The listing builds one solid part. Answer for the finished solid, in the listing's coordinates (mm). Round coordinates to 2 decimals unless told otherwise and drop trailing zeros. Write each loop counter-clockwise with the first axis right and the second up, starting at its lowest first coordinate (ties: lowest second). Pieces come first, ordered by that corner, then holes.
(1) A cutting plane is placed at A-A, the plane y = 0. Give the vertices of the cut face in (x, z), and give its area (3 significant figures).
(2) A cutting plane is placed at D-D, the plane z = 1.1. Give the number of separate pieces and of enclosed holes in the cut face, and give its area (3 significant figures).
(3) Each of these flat-tipped pins is pushed along its axis until it touches: pin 1 Ø1 at (x, z) = (22, 0.5) entering from +Y; pin 2 Ø3.5 at (x, y) = (-52.5, 0) entering from +Z. Where does it stop, or does it pass through?
(4) A cutting plane is placed at C-C, the plane y = 31.5. Give the vertices of the cut face in (x, z), and give its area (3 significant figures).
(5) Find the intervals of material crossed by probe 1 along Y at (x, z) = (-38, 1.4); probe 2 along Y at (x, z) = (19.5, 1.55); probe 3 along X at (y, z) = (25, 1.8), in increasing order.
from build123d import *

# Parameters (mm, degrees)
SKETCH_1_R          = 75
SKETCH_1_R_2        = 2
SKETCH_1_R_3        = 46
EXTRUDE_1_DEPTH     = 2
CUT_EXTRUDE_2_DEPTH = 10
SKETCH_5_R          = 1.65
CUT_EXTRUDE_3_DEPTH = 10
FILLET_2_R          = 2


with BuildPart() as part:
    # 草图1 → 凸台-拉伸1 (new body)
    with BuildSketch(Plane.XY):
        Circle(SKETCH_1_R)
        with Locations((-52.5, 0)):
            Circle(SKETCH_1_R_2, mode=Mode.SUBTRACT)
        with Locations((0, 52.5)):
            Circle(SKETCH_1_R_2, mode=Mode.SUBTRACT)
        with Locations((52.5, 0)):
            Circle(SKETCH_1_R_2, mode=Mode.SUBTRACT)
        with Locations((0, -52.5)):
            Circle(SKETCH_1_R_2, mode=Mode.SUBTRACT)
        Circle(SKETCH_1_R_3, mode=Mode.SUBTRACT)
    extrude(amount=EXTRUDE_1_DEPTH)

    # 草图3 → 切除-拉伸2 (cut)
    with BuildSketch(Plane.XY.offset(2)):
        with BuildLine():
            Line((-51.775970298, -18.553945664), (-61.172994758, -21.974182859))
            ThreePointArc((-61.172994758, -21.974182859), (-46.153503513, -45.769576287), (-22.484399296, -60.98730842))
            Line((-22.484399296, -60.98730842), (-19.064163111, -51.59028673))
            ThreePointArc((-19.064163111, -51.59028673), (-39.082362813, -38.698435587), (-51.775970298, -18.553945664))
        make_face()
        with BuildLine():
            Line((51.775970298, 18.553945664), (61.172994758, 21.974182859))
            ThreePointArc((61.172994758, 21.974182859), (46.153503513, 45.769576287), (22.484399296, 60.98730842))
            Line((22.484399296, 60.98730842), (19.064163111, 51.59028673))
            ThreePointArc((19.064163111, 51.59028673), (39.082362813, 38.698435587), (51.775970298, 18.553945664))
        make_face()
    extrude(amount=-CUT_EXTRUDE_2_DEPTH, mode=Mode.SUBTRACT)

    # 草图5 → 切除-拉伸3 (cut)
    with BuildSketch(Plane.XY.offset(2)):
        with Locations((-63.53412763, 21.527067294)):
            Circle(SKETCH_5_R)
        with Locations((-42.216475186, 42.635304887)):
            Circle(SKETCH_5_R)
        with Locations((-20.898822743, 63.743542481)):
            Circle(SKETCH_5_R)
        with Locations((63.53412763, -21.527067294)):
            Circle(SKETCH_5_R)
        with Locations((42.216475186, -42.635304887)):
            Circle(SKETCH_5_R)
        with Locations((20.898822743, -63.743542481)):
            Circle(SKETCH_5_R)
    extrude(amount=-CUT_EXTRUDE_3_DEPTH, mode=Mode.SUBTRACT)

    # 圆角2
    fillet_2_edges = [part.edges().sort_by_distance(p)[0] for p in [
        (51.775970298, 18.553945664, 1),
        (19.064163111, 51.59028673, 1),
        (22.484399296, 60.98730842, 1),
        (61.172994758, 21.974182859, 1),
    ]]
    fillet(fillet_2_edges, radius=FILLET_2_R)


solid = part.part
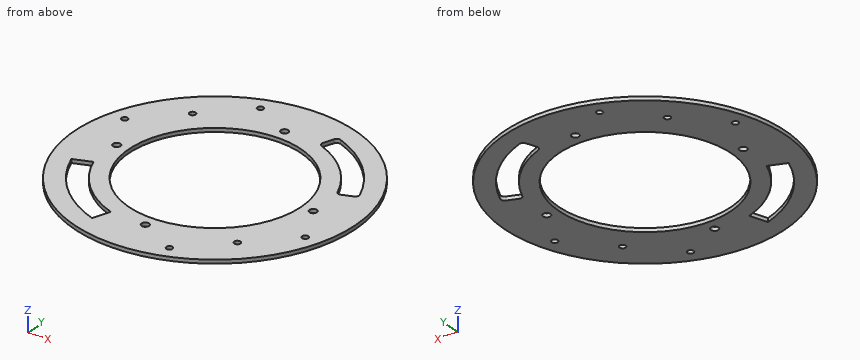
Solutions:
1. outline: (-75, 0) - (-54.5, 0) - (-54.5, 2) - (-75, 2) - close; (-50.5, 0) - (-46, 0) - (-46, 2) - (-50.5, 2) - close; (46, 0) - (50.5, 0) - (50.5, 2) - (46, 2) - close; (54.5, 0) - (75, 0) - (75, 2) - (54.5, 2) - close
1. area: 100 mm2
2. separate pieces: 1
2. enclosed holes: 13
2. area: 9,880 mm2
3. pin 1: stops at y = 71.85
3. pin 2: passes through
4. outline: (-68.06, 0) - (-33.52, 0) - (-33.52, 2) - (-68.06, 2) - close; (33.52, 0) - (45.09, 0) - (45.09, 2) - (33.52, 2) - close; (56.86, 0) - (68.06, 0) - (68.06, 2) - (56.86, 2) - close
4. area: 115 mm2
5. probe 1: y = -64.66 to -52.74, -39.76 to -25.92, 25.92 to 64.66
5. probe 2: y = -72.42 to -64.62, -62.87 to -41.66, 41.66 to 72.42
5. probe 3: x = -70.71 to -38.61, 38.61 to 48.99, 60 to 70.71
